Geometry check sheet. Reference: the model listing, model coordinates, mm. Round coordinates to 2 decimals unless told otherwise and drop trailing zeros. Loops run counter-clockwise (first coordinate to the right, second up) from the corner with the lowest first, then second, coordinate; pieces in that order, holes last. Notation, with made-up numbers: M 82.25,29 L 104.25,29 A29 cw 104.25,62 Z; hole C 55,51.5 d5. An arc over 180 degrees is marked long. Write item = value, one per line.
from build123d import *

# Parameters (mm, degrees)
PAD_DEPTH    = 0.245
POCKET_DEPTH = 0.05


with BuildPart() as part:
    # Sketch → Pad (new body, symmetric)
    with BuildSketch(Plane.XY):
        with BuildLine():
            Line((0, 0.375), (19.21, 0.375))
            ThreePointArc((19.21, -0.375), (19.585, 0), (19.21, 0.375))
            Line((19.21, -0.375), (0, -0.375))
            ThreePointArc((0, 0.375), (-0.375, 0), (0, -0.375))
        make_face()
    extrude(amount=PAD_DEPTH, both=True)

    # Sketch001 → Revolution (revolve)
    with BuildSketch(Plane.XY):
        with BuildLine():
            Line((0, 0.625), (0, 0))
            Line((0, 0), (0, -0.625))
            ThreePointArc((0, 0.625), (-0.625, 0), (0, -0.625))
        make_face()
    revolve(axis=Axis((0, 0, 0), (0, -1, 0)))

    # Sketch002 → Revolution001 (revolve)
    with BuildSketch(Plane.XY):
        with BuildLine():
            ThreePointArc((19.21, -0.625), (19.835, 0), (19.21, 0.625))
            Line((19.21, 0.625), (19.21, 0))
            Line((19.21, 0), (19.21, -0.625))
        make_face()
    revolve(axis=Axis((19.21, 0, 0), (0, -1, 0)))

    # Sketch003 (on DatumPlane) → Pocket (cut)
    with BuildSketch(Plane.XY.offset(0.25)):
        Polygon((1.05425, -0.16238), (1.148, 0), (1.05425, 0.16238), (0.86675, 0.16238), (0.773, 0), (0.86675, -0.16238), align=None)
    extrude(amount=-POCKET_DEPTH, mode=Mode.SUBTRACT)


solid = part.part
(1) Sectioned sample at A-A on x = 17. Record the cut outline in (y, z) (3 decimals).
Result set:
outline = M -0.375,-0.245 L 0.375,-0.245 L 0.375,0.245 L -0.375,0.245 Z
(2) Material ranges on line 1 along Z through (x, y) = (1, -0.3) (3 decimals); line 2 along Y through (x, z) = (12, -0.2) (3 decimals); line 3 along X through (y, z) = (-0.45, -0.2), recorded low to high. Write a range as from..to.
Result set:
line_1 = -0.245..0.245
line_2 = -0.375..0.375
line_3 = -0.38..0.38, 18.83..19.59
(3) Depth check by flat-ended pin: pin 1 Ø0.5 at (x, z) = (11.5, 0) entering from +Y (3 decimals). Enter the tip coordinate at first touch or a pass-through.
Result set:
pin_1 = 0.375
